Input: dimensioned drawing with shaded views. Units: mm. Origin: part minimum x, y, z. A direction names the side the tool comes from. Round coordinates to 2 decimals unless told otherwise and drop trailing zeros. Loops run counter-clockwise (first coordinate to the right, second up) from the corner with the lowest first, then second, coordinate; pieces in that order, holes last.
1) Section B-B, the plane z = 25. Return loops of the section in (x, y), and give its area (3 significant figures).
2) Access query for the marked faces 1 and 2. Directions: +Z, -Z, +X, -X, +Y, -Y. A direction counts if a zero-diameter tool reaches every point of the face in a straight line with its end or side. Return the directions, or none.
3) First-contact query: pin 1 (8 mm diameter, centred on x = 323.5, z = 17, fed in from +Y); pin 2 (4 mm diameter, centred on x = 65, y = 224.5, fed in from -Z); pin 3 (12 mm diameter, centred on x = 143.5, y = 80, fed in from +Z); pin 4 (1.5 mm diameter, centred on y = 315, z = 29, fed in from +X). Flat tips, straight axial feed; report the tip coordinate or a pass-through.
4) Section A-A, the plane y = 269.5. Return loops of the section in (x, z).
5) Ray query, line 1 along Y through (x, z) = (344, 30.5); line 2 along Z through (x, y) = (192.5, 269). Return the intervals inside material, ascending.
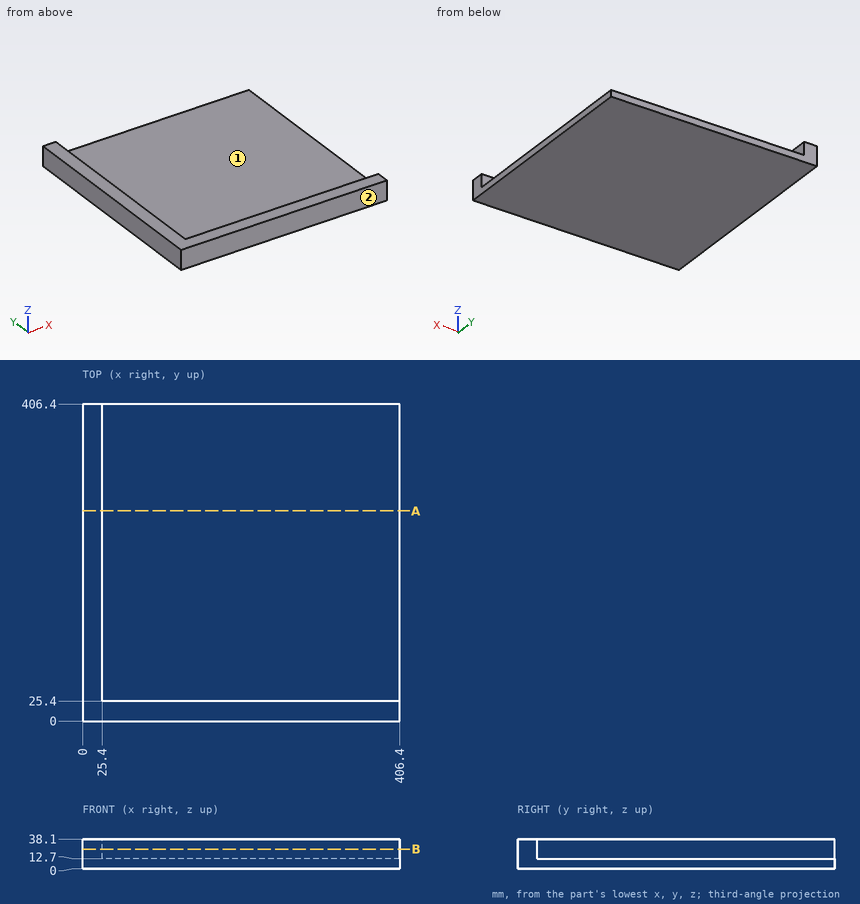
Final values:
1. outline: (0, 0) - (406.4, 0) - (406.4, 25.4) - (25.4, 25.4) - (25.4, 406.4) - (0, 406.4) - close
1. area: 20,000 mm2
2. face 1: +Z, +X, +Y
2. face 2: +Z, -Z, +X, -X, -Y
3. pin 1: stops at y = 25.4
3. pin 2: stops at z = 0
3. pin 3: stops at z = 12.7
3. pin 4: stops at x = 25.4
4. outline: (0, 0) - (406.4, 0) - (406.4, 12.7) - (25.4, 12.7) - (25.4, 38.1) - (0, 38.1) - close
5. line 1: y = 0 to 25.4
5. line 2: z = 0 to 12.7
